CAD build for the part. Positions are in the model's coordinates, mm. A direction names the side the tool comes from. Round coordinates to 2 decimals unless told otherwise and drop trailing zeros. Write each loop counter-clockwise with the first axis right and the second up, starting at its lowest first coordinate (ties: lowest second). Pieces come first, ordered by that corner, then holes. Notation, with made-up numbers: (74, 29) -> (103, 29) arc R20 ccw to (103, 37) -> close; hole circle Ø10 at (-38.5, 5). An arc over 180 degrees is marked (long way). Put each result on its own line as item: value. Start each with the question number.
1. Flat gauge pins, fed straight in: P1, Ø0.9, axis at x = 21, z = 3, coming from the +Y side; P2, Ø2, axis at x = -27.5, z = 4.5, coming from the -Y side. Where does each tip first touch, or does it go through?
2. Saw through at A-A on x = 0. List the corners of the cut face in (y, z), and give its area (3 significant figures).
3. Pull direction X, two halves, no side cores. Call faces 1 (the cylindrical face through (-1.08, -4.88, 2.48)), 2 (the cylindrical face through (38.1, -19.14, 1.51)), 3 (the cylindrical face through (-38.14, -0.24, 4.1)): pulls with the +X half, pulls with the -X half, needs draft (parallel to the pull), parting line crosses it, or undercut.
4. 3-axis set-ups, long thin cutter, end or side, ignore diameter. For faces 4 (the flat face through (-22, 11.5, 2)), 5 (the cylindrical face through (-38.14, 19.1, 1.51)): which of +Z, -Z, +X, -X, +Y, -Y reach the whole face in a straight line?
5. Drill centre lines: line 1 (X direction, y = 7.5, z = 0.55); line 2 (Y direction, x = 33.5, z = 1.4); line 3 (X direction, y = -4.5, z = 4.45). Where is each one in solid material? Low to high. Write a range as from..to.
6. Saw through at B-B on y = -10.5. List the corners of the cut face in (x, z).
7. Saw through at D-D on y = 0. State how many separate pieces and enclosed holes the cut face has, and give its area (3 significant figures).
8. Saw through at C-C on x = 33.5. List the corners of the cut face in (y, z), and give its area (3 significant figures).
from build123d import *

# Parameters (mm, degrees)
F0_R     = 1.5
F0_W     = 13.5
F0_H     = 23
F0_R_2   = 5
F1_DEPTH = 5
F2_R     = 3
F3_R     = 1
F4_R     = 1


with BuildPart() as f1:
    # F0 (on Top) → F1 (new body)
    with BuildSketch(Plane.XY):
        Polygon((0, 20), (-39, 20), (-39, -20), (39, -20), (39, 0), (39, 20), align=None)
        with Locations((-33.5, 0)):
            Circle(F0_R, mode=Mode.SUBTRACT)
        with Locations((-22.25, 0)):
            Rectangle(F0_W, F0_H, mode=Mode.SUBTRACT)
        Circle(F0_R_2, mode=Mode.SUBTRACT)
        Polygon((15.5, 11.5), (29, 11.5), (29, 0), (29, -11.5), (15.5, -11.5), align=None, mode=Mode.SUBTRACT)
        with Locations((33.5, 0)):
            Circle(F0_R, mode=Mode.SUBTRACT)
    extrude(amount=F1_DEPTH)

    # F2
    f2_edges = [f1.edges().sort_by_distance(p)[0] for p in [
        (0, 20, 5),
        (-39, 0, 5),
        (0, -20, 5),
        (39, 0, 5),
        (-39, -20, 2.5),
        (-39, 20, 2.5),
        (39, 20, 2.5),
        (39, -20, 2.5),
    ]]
    fillet(f2_edges, radius=F2_R)

    # F3
    f3_edges = [f1.edges().sort_by_distance(p)[0] for p in [
        (0, -20, 0),
    ]]
    fillet(f3_edges, radius=F3_R)

    # F4
    f4_edges = [f1.edges().sort_by_distance(p)[0] for p in [
        (-22.25, -11.5, 5),
        (-15.5, 0, 5),
        (-22.25, 11.5, 5),
        (-29, 0, 5),
        (15.5, 0, 5),
        (22.25, 11.5, 5),
        (29, 0, 5),
        (22.25, -11.5, 5),
        (-29, 0, 0),
        (-15.5, 0, 0),
        (-22.25, 11.5, 0),
        (-22.25, -11.5, 0),
        (22.25, -11.5, 0),
        (29, 0, 0),
        (22.25, 11.5, 0),
        (15.5, 0, 0),
        (-5, 0, 5),
        (-5, 0, 0),
    ]]
    fillet(f4_edges, radius=F4_R)


solid = f1.part
Return value:
1. P1: stops at y = 19.95
1. P2: stops at y = -19.6
2. outline: (-20, 1) arc R1 ccw to (-19, 0) -> (-6, 0) arc R1 ccw to (-5, 1) -> (-5, 4) arc R1 ccw to (-6, 5) -> (-17, 5) arc R3 ccw to (-20, 2) -> close; (5, 1) arc R1 ccw to (6, 0) -> (19, 0) arc R1 ccw to (20, 1) -> (20, 2) arc R3 ccw to (17, 5) -> (6, 5) arc R1 ccw to (5, 4) -> close
2. area: 145 mm^2
3. face 1: undercut
3. face 2: pulls with the +X half
3. face 3: pulls with the -X half
4. face 4: +Z, -Z
4. face 5: +Z, -Z, -X, +Y
5. line 1: x = -38.89..-29.11, -15.39..15.39, 29.11..38.89
5. line 2: y = -20..-1.5, 1.5..20
5. line 3: x = -37.73..-29.11, -15.39..-2.41, 2.41..15.39, 29.11..37.73
6. outline: (-39, 1) arc R1 ccw to (-38, 0) -> (-30, 0) arc R1 ccw to (-29, 1) -> (-29, 4) arc R1 ccw to (-30, 5) -> (-36, 5) arc R3 ccw to (-39, 2) -> close; (-15.5, 1) arc R1 ccw to (-14.5, 0) -> (14.5, 0) arc R1 ccw to (15.5, 1) -> (15.5, 4) arc R1 ccw to (14.5, 5) -> (-14.5, 5) arc R1 ccw to (-15.5, 4) -> close; (29, 1) arc R1 ccw to (30, 0) -> (38, 0) arc R1 ccw to (39, 1) -> (39, 2) arc R3 ccw to (36, 5) -> (30, 5) arc R1 ccw to (29, 4) -> close
7. separate pieces: 6
7. enclosed holes: 0
7. area: 168 mm^2
8. outline: (-20, 1) arc R1 ccw to (-19, 0) -> (-1.5, 0) -> (-1.5, 5) -> (-17, 5) arc R3 ccw to (-20, 2) -> close; (1.5, 0) -> (19, 0) arc R1 ccw to (20, 1) -> (20, 2) arc R3 ccw to (17, 5) -> (1.5, 5) -> close
8. area: 181 mm^2
